```python
from build123d import *

# Parameters (mm, degrees)
SKETCH1_W           = 38.1
SKETCH1_H           = 38.1
BOSS_EXTRUDE1_DEPTH = 2.54
SKETCH2_W           = 1.905
SKETCH2_H           = 38.1
BOSS_EXTRUDE2_DEPTH = 16.51
FILLET3_R           = 1.016


with BuildPart() as part:
    # Sketch1 → Boss-Extrude1 (new body)
    with BuildSketch(Plane(origin=(0, 0, 0), x_dir=(1, 0, 0), z_dir=(0, 1, 0))):
        Rectangle(SKETCH1_W, SKETCH1_H)
    extrude(amount=BOSS_EXTRUDE1_DEPTH)

    # Sketch2 → Boss-Extrude2 (add)
    with BuildSketch(Plane(origin=(0, 2.54, 0), x_dir=(1, 0, 0), z_dir=(0, 1, 0))):
        with Locations((-18.0975, 0)):
            Rectangle(SKETCH2_W, SKETCH2_H)
        with Locations((-14.478, 0.002613699)):
            Rectangle(SKETCH2_W, SKETCH2_H)
        with Locations((-10.8585, 0.005227397)):
            Rectangle(SKETCH2_W, SKETCH2_H)
        with Locations((-7.239, 0.007841096)):
            Rectangle(SKETCH2_W, SKETCH2_H)
        with Locations((-3.6195, 0.010454795)):
            Rectangle(SKETCH2_W, SKETCH2_H)
        with Locations((0, 0.013068494)):
            Rectangle(SKETCH2_W, SKETCH2_H)
        with Locations((3.6195, 0.015682192)):
            Rectangle(SKETCH2_W, SKETCH2_H)
        with Locations((7.239, 0.018295891)):
            Rectangle(SKETCH2_W, SKETCH2_H)
        with Locations((10.8585, 0.02090959)):
            Rectangle(SKETCH2_W, SKETCH2_H)
        with Locations((14.478, 0.023523288)):
            Rectangle(SKETCH2_W, SKETCH2_H)
        with Locations((18.0975, 0.026136987)):
            Rectangle(SKETCH2_W, SKETCH2_H)
    extrude(amount=BOSS_EXTRUDE2_DEPTH)

    # Fillet3
    # the kernel refuses this fillet: 1.016 mm, written as the material it takes off along each edge
    with BuildSketch(Plane(origin=(-19.05, 19.05, 21.59), x_dir=(1, 0, 0), z_dir=(0, 0, -1)), Plane(origin=(17.145, 19.05, -21.616136987), x_dir=(0, -1, 0), z_dir=(0, 0, 1)), Plane(origin=(13.5255, 19.05, -21.613523288), x_dir=(0, -1, 0), z_dir=(0, 0, 1)), Plane(origin=(9.906, 19.05, -21.61090959), x_dir=(0, -1, 0), z_dir=(0, 0, 1)), Plane(origin=(6.2865, 19.05, -21.608295891), x_dir=(0, -1, 0), z_dir=(0, 0, 1)), Plane(origin=(2.667, 19.05, -21.605682192), x_dir=(0, -1, 0), z_dir=(0, 0, 1)), Plane(origin=(-0.9525, 19.05, -21.603068494), x_dir=(0, -1, 0), z_dir=(0, 0, 1)), Plane(origin=(-4.572, 19.05, -21.600454795), x_dir=(0, -1, 0), z_dir=(0, 0, 1)), Plane(origin=(-8.1915, 19.05, -21.597841096), x_dir=(0, -1, 0), z_dir=(0, 0, 1)), Plane(origin=(-11.811, 19.05, -21.595227397), x_dir=(0, -1, 0), z_dir=(0, 0, 1)), Plane(origin=(-15.4305, 19.05, -21.592613699), x_dir=(0, -1, 0), z_dir=(0, 0, 1))) as fillet3_piece_1:
        with BuildLine():
            CenterArc((FILLET3_R, FILLET3_R), FILLET3_R, 180, 90)
            Line((0, FILLET3_R), (0, 0))
            Line((0, 0), (FILLET3_R, 0))
        make_face()
    extrude(amount=43.18, mode=Mode.SUBTRACT)
    with BuildSketch(Plane(origin=(-17.145, 19.05, -21.59), x_dir=(0, -1, 0), z_dir=(0, 0, 1)), Plane(origin=(19.05, 19.05, 21.563863013), x_dir=(-1, 0, 0), z_dir=(0, 0, -1)), Plane(origin=(15.4305, 19.05, 21.566476712), x_dir=(-1, 0, 0), z_dir=(0, 0, -1)), Plane(origin=(11.811, 19.05, 21.56909041), x_dir=(-1, 0, 0), z_dir=(0, 0, -1)), Plane(origin=(8.1915, 19.05, 21.571704109), x_dir=(-1, 0, 0), z_dir=(0, 0, -1)), Plane(origin=(4.572, 19.05, 21.574317808), x_dir=(-1, 0, 0), z_dir=(0, 0, -1)), Plane(origin=(0.9525, 19.05, 21.576931506), x_dir=(-1, 0, 0), z_dir=(0, 0, -1)), Plane(origin=(-2.667, 19.05, 21.579545205), x_dir=(-1, 0, 0), z_dir=(0, 0, -1)), Plane(origin=(-6.2865, 19.05, 21.582158904), x_dir=(-1, 0, 0), z_dir=(0, 0, -1)), Plane(origin=(-9.906, 19.05, 21.584772603), x_dir=(-1, 0, 0), z_dir=(0, 0, -1)), Plane(origin=(-13.5255, 19.05, 21.587386301), x_dir=(-1, 0, 0), z_dir=(0, 0, -1))) as fillet3_piece_2:
        with BuildLine():
            CenterArc((FILLET3_R, -FILLET3_R), FILLET3_R, 90, 90)
            Line((0, -FILLET3_R), (0, 0))
            Line((0, 0), (FILLET3_R, 0))
        make_face()
    extrude(amount=43.18, mode=Mode.SUBTRACT)


solid = part.part
```
Build history of the part. All positions in model axes, mm. Coordinates: 2 decimals unless noted, no trailing zeros. Write each loop counter-clockwise with the first axis right and the second up, starting at its lowest first coordinate (ties: lowest second). Pieces come first, ordered by that corner, then holes.
1. Drill centre lines: probe 1 along Y at (x, z) = (3.5, -8); probe 2 along Z at (x, y) = (-10, 12); probe 3 along Y at (x, z) = (-17, 7). Where is each one in solid material? Low to high.
Answer block:
probe 1: y = 0 to 19.03
probe 2: z = -19.06 to 19.04
probe 3: y = 0 to 2.54
2. Band-saw the part on A-A, the plane y = 16.25. Give the number of separate pieces and of enclosed holes in the cut face, and give its area (3 significant figures).
Answer block:
separate pieces: 11
enclosed holes: 0
area: 798 mm2
3. Band-saw the part on B-B, the plane x = -1.5. Give the cut face in (y, z).
Answer block:
outline: (0, -19.05) - (2.54, -19.05) - (2.54, 19.05) - (0, 19.05) - close
4. Pull direction X, two halves, no side cores. Call faces 1 (the cylindrical face through (0.67, 18.737, 0.254)), 2 (the flat face through (-19.05, 9, 0)), 3 (the flat face through (9, 2.54, 0)), 4 (the flat face through (-3, 2, 19.05)): released by +X, released by -X, zero draft, split by the parting line, or undercut.
Answer block:
face 1: undercut
face 2: released by -X
face 3: undercut
face 4: zero draft
5. Drop flat-ended pins along their axis: pin 1 (1 mm diameter, centred on x = -11, y = 8.5, fed in from -Z); pin 2 (3 mm diameter, centred on x = 13.5, y = 6.5, fed in from +Z); pin 3 (1.5 mm diameter, centred on x = -8.5, z = 15, fed in from +Y). Give the stop position or say it passes through.
Answer block:
pin 1: stops at z = -19.06
pin 2: stops at z = 19.03
pin 3: stops at y = 18.87
